```python
from build123d import *

# Parameters (mm, degrees)
CUT_EXTRUDE1_DEPTH      = 59.159460492
CUT_EXTRUDE1_DEPTH_BACK = 59.159460492
SKETCH3_R               = 4


with BuildPart() as part:
    # Sketch2 → Revolve1 (revolve)
    with BuildSketch(Plane(origin=(0, 0, 0), x_dir=(0, 0, -1), z_dir=(1, 0, 0)), mode=Mode.PRIVATE) as revolve1_sk:
        with BuildLine():
            Line((-10, 4), (10, 4))
            ThreePointArc((10, 4), (24.92820323, 0), (10, -4))
            Line((10, -4), (-10, -4))
            Line((-10, -4), (-10, 4))
        make_face()
    revolve(revolve1_sk.sketch.rotate(Axis((0, 4, 10), (0, -1, 0)), 180), axis=Axis((0, 4, 10), (0, -1, 0)))

    # Sketch3 → Cut-Extrude1 (cut, two sides: drawn at the far end of the back side and taken through both)
    with BuildSketch(Plane(origin=(0, 4, 0), x_dir=(1, 0, 0), z_dir=(0, 1, 0)).offset(-CUT_EXTRUDE1_DEPTH_BACK)):
        with Locations(Location((-8, -2, 0), (0, 0, 90))):
            Circle(SKETCH3_R)
        with Locations(Location((8, -2, 0), (0, 0, 90))):
            Circle(SKETCH3_R)
        with Locations(Location((8, -18, 0), (0, 0, 90))):
            Circle(SKETCH3_R)
        with Locations(Location((-8, -18, 0), (0, 0, 90))):
            Circle(SKETCH3_R)
    extrude(amount=CUT_EXTRUDE1_DEPTH + CUT_EXTRUDE1_DEPTH_BACK, mode=Mode.SUBTRACT)


solid = part.part
```
Read the model definition and answer for the solid it produces. Units are mm, in the model's axes. A direction names the side the tool comes from. Round coordinates to 2 decimals unless told otherwise and drop trailing zeros. Write each loop counter-clockwise with the first axis right and the second up, starting at its lowest first coordinate (ties: lowest second). Pieces come first, ordered by that corner, then holes. Notation, with made-up numbers: (49.25, -29.5) -> (78.25, -29.5) arc R37 cw to (78.25, 8.5) -> close; hole circle Ø5 at (65, -19). An arc over 180 degrees is marked (long way). Answer in a Markdown table with one row per item. Add a question column.
1) Find section D-D, the plane y = -5.5. Determine the outline of the cut face in (x, z).
2) Which of the six approach directions +Z, -Z, +X, -X, +Y, -Y give full straight-line access (tool end or side, diameter ignored) to faces 1 (the face through (0, 4, 10)), 2 (the face through (-4.095, -0.056, 2.867)), 3 (the face through (0, -4, 10))?
3) Find section B-B, the plane x = -8. State how many separate pieces and enclosed holes the cut face has, and give its area (3 significant figures).
4) Given P1, Ø9, axis at x = -8, z = 2, coming from the +Y side; P2, Ø2, axis at x = 21.5, z = 18, coming from the +Y side; P3, Ø13, axis at x = 8, z = 2, coming from the -Y side; P4, Ø10, axis at x = -9.5, z = -11.5, coming from the -Y side, each flat-ended and moving along its own axis, determine where each tip first touches the part or whether it passes through.
5) Consider line 1 (X direction, y = -0.5, z = 2); line 2 (X direction, y = -1, z = 2); line 3 (X direction, y = -6, z = -1.5). Determine where each line is inside the solid, lowest interval first.
6) Find section A-A, the plane y = 0.25. Determine the outline of the cut face in (x, z), and give its area (3 significant figures).
Findings below:
| question | item | result |
|---|---|---|
| 1 | outline | circle Ø65.48 at (0, 10); hole circle Ø42.24 at (0, 10) |
| 2 | face 1 | +Y |
| 2 | face 2 | +Y, -Y |
| 2 | face 3 | -Y |
| 3 | separate pieces | 3 |
| 3 | enclosed holes | 0 |
| 3 | area | 575 mm² |
| 4 | P1 | y = 4 |
| 4 | P2 | y = 7.42 |
| 4 | P3 | y = -4 |
| 4 | P4 | y = -8 |
| 5 | line 1 | -33.98 to -12, -4 to 4, 12 to 33.98 |
| 5 | line 2 | -33.94 to -12, -4 to 4, 12 to 33.94 |
| 5 | line 3 | -30.1 to -18.33, 18.33 to 30.1 |
| 6 | outline | circle Ø69.85 at (0, 10); hole circle Ø8 at (-8, 2); hole circle Ø8 at (-8, 18); hole circle Ø8 at (8, 2); hole circle Ø8 at (8, 18) |
| 6 | area | 3,630 mm² |
